CAD build for the part. Positions are in the model's coordinates, mm. Round coordinates to 2 decimals unless told otherwise and drop trailing zeros. Order: outer loops, then holes, each group sorted by start corner. A loop starts at its lowest first (then second) coordinate and runs counter-clockwise, first axis right, second up. Notation, with made-up numbers: M 16,83 L 39,83 A29 ccw 39,112 Z; hole C -40,44.25 d1. An arc over 180 degrees is marked long. Answer as a JSON object with one key per item and string values.
```python
from build123d import *

# Parameters (mm, degrees)
SKETCH1_W           = 10
SKETCH1_H           = 40
BOSS_EXTRUDE1_DEPTH = 10
SKETCH3_R           = 2
CUT_EXTRUDE2_DEPTH  = 43.426406871


with BuildPart() as part:
    # Sketch1 → Boss-Extrude1 (new body)
    with BuildSketch(Plane.XY):
        with Locations((5, 20)):
            Rectangle(SKETCH1_W, SKETCH1_H)
    extrude(amount=BOSS_EXTRUDE1_DEPTH)

    # Sketch3 → Cut-Extrude2 (cut, through all)
    with BuildSketch(Plane.ZY):
        with Locations((5, 35)):
            Circle(SKETCH3_R)
        with Locations(Location((5, 5, 0), (0, 0, 180))):
            Circle(SKETCH3_R)
    extrude(amount=-CUT_EXTRUDE2_DEPTH, mode=Mode.SUBTRACT)


solid = part.part
```
Item 1: Saw through at B-B on y = 35. List the corners of the cut face in (x, z), and give its area (3 significant figures).
Worked answers:
{"outline": "M 0,0 L 10,0 L 10,3 L 0,3 Z; M 0,7 L 10,7 L 10,10 L 0,10 Z", "area": "60.0 mm2"}
Item 2: Wall check: line 1 along Y through (x, z) = (2.25, 5); line 2 along Y through (x, z) = (8, 3.25); line 3 along Z through (x, y) = (6.25, 5). Give the ranges that are in metal, low to high. Write a range as [from, to].
Worked answers:
{"line 1": "y = [0, 3], [7, 33], [37, 40]", "line 2": "y = [0, 4.03], [5.97, 34.03], [35.97, 40]", "line 3": "z = [0, 3], [7, 10]"}
Item 3: Saw through at D-D on y = 5.5. List the corners of the cut face in (x, z).
Worked answers:
{"outline": "M 0,0 L 10,0 L 10,3.06 L 0,3.06 Z; M 0,6.94 L 10,6.94 L 10,10 L 0,10 Z"}
Item 4: Saw through at C-C on x = 8.5. List the corners of the cut face in (y, z).
Worked answers:
{"outline": "M 0,0 L 40,0 L 40,10 L 0,10 Z; hole C 5,5 d4; hole C 35,5 d4"}
Item 5: Two-plate mould, pull along Y, no slides. Class faces 1 (the flat face through (5, 0, 5)), 2 (the cylindrical face through (5, 33, 5)), 3 (the flat face through (0, 20, 5)): released by +Y, released by -Y, zero draft, split by the parting line, or undercut.
Worked answers:
{"face 1": "released by -Y", "face 2": "undercut", "face 3": "zero draft"}
Item 6: Drop a flat-ended pin along its axis: pin 1 Ø1 at (y, z) = (4, 5) entering from -X. Give the stop position or say it passes through.
Worked answers:
{"pin 1": "passes through"}
Item 7: Saw through at A-A on z = 5. List the corners of the cut face in (x, y).
Worked answers:
{"outline": "M 0,0 L 10,0 L 10,3 L 0,3 Z; M 0,7 L 10,7 L 10,33 L 0,33 Z; M 0,37 L 10,37 L 10,40 L 0,40 Z"}
